Could you check a few things on this model? Use its own coordinates, in mm. Face numbers are marked on the shaded views. A direction names the side the tool comes from. Give positions to 0.01 mm unless a question says otherwise; leave off trailing zeros. Write each loop counter-clockwise with the first axis right and the second up, starting at its lowest first coordinate (ties: lowest second). Pieces come first, ordered by that corner, then holes. Notation, with made-up numbers: (0, 56) -> (49, 56) arc R16 cw to (49, 69) -> close; hole circle Ø7 at (59, 80). An arc over 180 degrees is marked (long way). One line per question, with ' | ' between items.
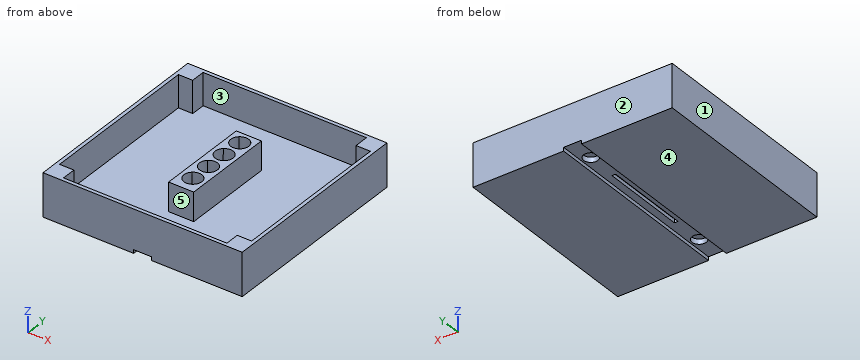
from build123d import *

# Parameters (mm, degrees)
SKICA1_W                 = 55.6
SKICA1_H                 = 55.6
P_IDAT_VYSUNUT_M1_DEPTH  = 3
SKICA2_W                 = 5
SKICA2_H                 = 55.6
ODEBRAT_VYSUNUT_M1_DEPTH = 1
SKICA3_R                 = 2
SKICA3_W                 = 1
SKICA3_H                 = 24
ODEBRAT_VYSUNUT_M2_DEPTH = 1.4
SKICA4_W                 = 7
SKICA4_H                 = 26
P_IDAT_VYSUNUT_M2_DEPTH  = 8
LINPOLE1_COUNT           = 4
LINPOLE1_PITCH           = 6
SKICA9_W                 = 54.6
SKICA9_H                 = 1
SKICA9_W_2               = 1
SKICA9_H_2               = 53.6
SKICA9_W_3               = 4
SKICA9_H_3               = 4
P_IDAT_VYSUNUT_M3_DEPTH  = 9


with BuildPart() as part:
    # Skica1 → Přidat vysunutím1 (new body)
    with BuildSketch(Plane.XY):
        Rectangle(SKICA1_W, SKICA1_H)
    extrude(amount=P_IDAT_VYSUNUT_M1_DEPTH)

    # Skica2 → Odebrat vysunutím1 (cut)
    with BuildSketch(Plane(origin=(0, 0, 0), x_dir=(-1, 0, 0), z_dir=(0, 0, -1))):
        Rectangle(SKICA2_W, SKICA2_H)
    extrude(amount=-ODEBRAT_VYSUNUT_M1_DEPTH, mode=Mode.SUBTRACT)

    # Skica3 → Odebrat vysunutím2 (cut)
    with BuildSketch(Plane(origin=(0, 0, 1), x_dir=(-1, 0, 0), z_dir=(0, 0, -1))):
        with Locations((0, 20.8)):
            Circle(SKICA3_R)
        with Locations((0, -20.8)):
            Circle(SKICA3_R)
        Rectangle(SKICA3_W, SKICA3_H)
    extrude(amount=-ODEBRAT_VYSUNUT_M2_DEPTH, mode=Mode.SUBTRACT)

    # Skica4 → Přidat vysunutím2 (add)
    with BuildSketch(Plane.XY.offset(3)):
        Rectangle(SKICA4_W, SKICA4_H)
    extrude(amount=P_IDAT_VYSUNUT_M2_DEPTH)

    # Odebrat spojením profilů2: read off the stored shape, not the designer's step
    # Odebrat spojením profilů2: loft between two sections, ruled curve by curve
    odebrat_spojen_m_profil_2_from = [
        Edge.make_bspline([(-2.5, 6.525099132, 2), (-2.083333333, 6.525099132, 2), (-1.666666667, 6.525099132, 2), (-0.833333333, 6.525099132, 2), (-0.416666667, 6.525099132, 2), (0.416666667, 6.525099132, 2), (0.833333333, 6.525099132, 2), (1.666666667, 6.525099132, 2), (2.083333333, 6.525099132, 2), (2.5, 6.525099132, 2)], [0, 0, 0, 0, 0.25, 0.25, 0.5, 0.5, 0.75, 0.75, 1, 1, 1, 1], 3),
        Edge.make_bspline([(-2.5, 12.474900868, 2), (-2.5, 11.979084057, 2), (-2.5, 11.483267245, 2), (-2.5, 10.491633623, 2), (-2.5, 9.995816811, 2), (-2.5, 9.004183189, 2), (-2.5, 8.508366377, 2), (-2.5, 7.516732755, 2), (-2.5, 7.020915943, 2), (-2.5, 6.525099132, 2)], [0, 0, 0, 0, 0.25, 0.25, 0.5, 0.5, 0.75, 0.75, 1, 1, 1, 1], 3),
        Edge.make_bspline([(2.5, 12.474900868, 2), (2.083333333, 12.474900868, 2), (1.666666667, 12.474900868, 2), (0.833333333, 12.474900868, 2), (0.416666667, 12.474900868, 2), (-0.416666667, 12.474900868, 2), (-0.833333333, 12.474900868, 2), (-1.666666667, 12.474900868, 2), (-2.083333333, 12.474900868, 2), (-2.5, 12.474900868, 2)], [0, 0, 0, 0, 0.25, 0.25, 0.5, 0.5, 0.75, 0.75, 1, 1, 1, 1], 3),
        Edge.make_bspline([(2.5, 6.525099132, 2), (2.5, 7.020915943, 2), (2.5, 7.516732755, 2), (2.5, 8.508366377, 2), (2.5, 9.004183189, 2), (2.5, 9.995816811, 2), (2.5, 10.491633623, 2), (2.5, 11.483267245, 2), (2.5, 11.979084057, 2), (2.5, 12.474900868, 2)], [0, 0, 0, 0, 0.25, 0.25, 0.5, 0.5, 0.75, 0.75, 1, 1, 1, 1], 3),
    ]
    odebrat_spojen_m_profil_2_to = [
        Edge.make_bspline([(-1.608388791, 7.586081116, 11), (-1.403167079, 7.413620149, 11), (-1.156724267, 7.264297071, 11), (-0.606690103, 7.056988388, 11), (-0.303658501, 7, 11), (0.303658501, 7, 11), (0.606690103, 7.056988388, 11), (1.156724267, 7.264297071, 11), (1.403167079, 7.413620149, 11), (1.608388791, 7.586081116, 11)], [0, 0, 0, 0, 0.25, 0.25, 0.5, 0.5, 0.75, 0.75, 1, 1, 1, 1], 3),
        Edge.make_bspline([(-1.608388791, 11.413918884, 11), (-1.852594491, 11.208697172, 11), (-2.079966955, 10.935038102, 11), (-2.405399483, 10.274370851, 11), (-2.5, 9.8882136, 11), (-2.5, 9.1117864, 11), (-2.405399483, 8.725629149, 11), (-2.079966955, 8.064961898, 11), (-1.852594491, 7.791302828, 11), (-1.608388791, 7.586081116, 11)], [0, 0, 0, 0, 0.25, 0.25, 0.5, 0.5, 0.75, 0.75, 1, 1, 1, 1], 3),
        Edge.make_bspline([(1.608388791, 11.413918884, 11), (1.403167079, 11.586379851, 11), (1.156724267, 11.735702929, 11), (0.606690103, 11.943011612, 11), (0.303658501, 12, 11), (-0.303658501, 12, 11), (-0.606690103, 11.943011612, 11), (-1.156724267, 11.735702929, 11), (-1.403167079, 11.586379851, 11), (-1.608388791, 11.413918884, 11)], [0, 0, 0, 0, 0.25, 0.25, 0.5, 0.5, 0.75, 0.75, 1, 1, 1, 1], 3),
        Edge.make_bspline([(1.608388791, 7.586081116, 11), (1.852594491, 7.791302828, 11), (2.079966955, 8.064961898, 11), (2.405399483, 8.725629149, 11), (2.5, 9.1117864, 11), (2.5, 9.8882136, 11), (2.405399483, 10.274370851, 11), (2.079966955, 10.935038102, 11), (1.852594491, 11.208697172, 11), (1.608388791, 11.413918884, 11)], [0, 0, 0, 0, 0.25, 0.25, 0.5, 0.5, 0.75, 0.75, 1, 1, 1, 1], 3),
    ]
    odebrat_spojen_m_profil_2 = Solid(Shell([*[Face.make_surface_from_curves(odebrat_spojen_m_profil_2_from[k], odebrat_spojen_m_profil_2_to[k]) for k in range(4)], Face(Wire(odebrat_spojen_m_profil_2_from)), Face(Wire(odebrat_spojen_m_profil_2_to))]))
    add(odebrat_spojen_m_profil_2, mode=Mode.SUBTRACT)

    # LinPole1: Odebrat spojením profilů2 ×4
    with Locations(*[(0, -i * LINPOLE1_PITCH, 0) for i in range(1, LINPOLE1_COUNT)]):
        add(odebrat_spojen_m_profil_2, mode=Mode.SUBTRACT)

    # Skica9 → Přidat vysunutím3 (add)
    with BuildSketch(Plane.XY.offset(3)):
        Polygon((-26.8, 22.8), (-26.8, 26.8), (-26.8, 27.8), (-27.8, 27.8), (-27.8, -27.8), (-26.8, -27.8), (-26.8, -26.8), (-26.8, -22.8), align=None)
        Polygon((22.8, 26.8), (26.8, 26.8), (27.8, 26.8), (27.8, 27.8), (-26.8, 27.8), (-26.8, 26.8), (-22.8, 26.8), align=None)
        with Locations((0.5, -27.3)):
            Rectangle(SKICA9_W, SKICA9_H)
        with Locations((27.3, 0)):
            Rectangle(SKICA9_W_2, SKICA9_H_2)
        with Locations((-24.8, 24.8)):
            Rectangle(SKICA9_W_3, SKICA9_H_3)
        with Locations((24.8, 24.8)):
            Rectangle(SKICA9_W_3, SKICA9_H_3)
        with Locations((24.8, -24.8)):
            Rectangle(SKICA9_W_3, SKICA9_H_3)
        with Locations((-24.8, -24.8)):
            Rectangle(SKICA9_W_3, SKICA9_H_3)
    extrude(amount=P_IDAT_VYSUNUT_M3_DEPTH)


solid = part.part
Q1. On a 3-axis mill with a long thin cutter (end or side, diameter ignored), from which of +Z, -Z, +X, -X, +Y, -Y can I reach the whole of each face in a straight line? I mean the marked faces 4 and 5. Say none if no direction works.
Answer below:
face 4: -Z, +X, -X, +Y, -Y | face 5: +Z
Q2. If I drill on line 1 along Y through (x, z) = (0, 1.75); line 2 along Y through (x, z) = (0, 2.05); line 3 along X through (y, z) = (-1.5, 11.25), over which ranges is the centre line in solid material (lowest first)?
Answer below:
line 1: y = -27.8 to -22.8, -18.8 to -12, 12 to 18.8, 22.8 to 27.8 | line 2: y = -27.8 to -22.8, -18.8 to -12, 12.47 to 18.8, 22.8 to 27.8 | line 3: x = -27.8 to -26.8, 26.8 to 27.8
Q3. Imagine slicing it at B-B on z = 5.5. Count the separate pieces of the cut face and the enclosed holes in it, and give its area (3 significant figures).
Answer below:
separate pieces: 2 | enclosed holes: 5 | area: 362 mm^2
Q4. Imagine slicing it at C-C on y = 20.8. Please give me the cut outline in (x, z).
Answer below:
outline: (-27.8, 0) -> (-2.5, 0) -> (-2.5, 1) -> (-2, 1) -> (-2, 2.4) -> (2, 2.4) -> (2, 1) -> (2.5, 1) -> (2.5, 0) -> (27.8, 0) -> (27.8, 12) -> (26.8, 12) -> (26.8, 3) -> (-26.8, 3) -> (-26.8, 12) -> (-27.8, 12) -> close
Q5. Will these pins go through, and if not, where does the flat tip stop? pin 1 (0.6 mm diameter, centred on x = 1, y = -9, fed in from +Z); pin 2 (2.5 mm diameter, centred on x = 0, y = 20.8, fed in from -Z); pin 3 (12 mm diameter, centred on x = -3, y = 11.5, fed in from +Z); pin 4 (4 mm diameter, centred on x = 1, y = -3.5, fed in from -Z).
Answer below:
pin 1: stops at z = 2 | pin 2: stops at z = 2.4 | pin 3: stops at z = 11 | pin 4: stops at z = 0
Q6. If we mould it in two halves opening along Y, with no side actions, what happens to the marked faces 1, 2 and 3? For each: +Y half, -Y half, draft (parallel to the pull), parting line (faces both ways), or undercut.
Answer below:
face 1: draft | face 2: +Y half | face 3: undercut
Q7. Imagine slicing it at A-A on x = 12.5. Please give me the cut outline in (y, z), and give its area (3 significant figures).
Answer below:
outline: (-27.8, 0) -> (27.8, 0) -> (27.8, 12) -> (26.8, 12) -> (26.8, 3) -> (-26.8, 3) -> (-26.8, 12) -> (-27.8, 12) -> close | area: 185 mm^2
